Model file for the job. Use its own axes, mm. A direction names the side the tool comes from. Give positions to 0.01 mm unless a question says otherwise; leave off trailing zeros. Loops run counter-clockwise (first coordinate to the right, second up) from the corner with the lowest first, then second, coordinate; pieces in that order, holes last. Notation, with made-up numbers: (-34.5, 31.25) -> (24.5, 31.25) arc R12 cw to (24.5, 41.25) -> close; hole circle Ø4 at (38.5, 55). An arc over 180 degrees is marked (long way). Use CSV: the item, a comma, the result in double quotes. Start each with the question number.
(1) Flat gauge pins, fed straight in: pin 1 (1.8 mm diameter, centred on x = 0.5, z = -0.5, fed in from +Y); pin 2 (2 mm diameter, centred on y = 1, z = 1.5, fed in from +X); pin 3 (1 mm diameter, centred on y = 2, z = 1, fed in from -X). Where does each tip first touch, or does it go through?
(2) 3-axis set-ups, long thin cutter, end or side, ignore diameter. For faces 1 (the flat face through (2.39, 1.23, -1.36)), 2 (the cylindrical face through (1.01, 2.87, 2.45)): which of +Z, -Z, +X, -X, +Y, -Y reach the whole face in a straight line?
(3) Cut at A-A on y = 1.6. Write the cut outline in (x, z), then the cut area to 3 significant figures.
(4) Drill centre lines: probe 1 along X at (y, z) = (1.2, 0.1); probe 2 along Z at (x, y) = (-0.5, 1.1); probe 3 along Z at (x, y) = (1.25, 0.5). Where is each one in solid material? Low to high.
(5) Cut at C-C on y = 2.7. Write the cut outline in (x, z).
(6) Pull direction Z, two halves, no side cores. Call faces 3 (the flat face through (2.37, 1.234, 1.394)), 4 (the flat face through (0, 1, -2.75)), 5 (the flat face through (1.3, 0, -1.2)), 6 (the cylindrical face through (0.45, 1.97, 1.43)): pulls with the +Z half, pulls with the -Z half, needs draft (parallel to the pull), parting line crosses it, or undercut.
from build123d import *

# Parameters (mm, degrees)
SKETCH1_R           = 1.5
BOSS_EXTRUDE1_DEPTH = 4
FILLET1_R           = 0.1
CUT_EXTRUDE1_START  = -0.1
SKETCH3_R           = 1.8
SKETCH3_R_2         = 1.5
CUT_EXTRUDE1_DEPTH  = 0.1
FILLET2_R           = 0.1


with BuildPart() as part:
    # Sketch1 → Boss-Extrude1 (new body)
    with BuildSketch(Plane(origin=(0, 0, 0), x_dir=(1, 0, 0), z_dir=(0, 1, 0))):
        Polygon((1.58771324, -2.75), (3.175426481, 0), (1.58771324, 2.75), (-1.58771324, 2.75), (-3.175426481, 0), (-1.58771324, -2.75), align=None)
        with Locations(Location((0, 0, 0), (0, 0, 270))):
            Circle(SKETCH1_R, mode=Mode.SUBTRACT)
    extrude(amount=BOSS_EXTRUDE1_DEPTH)

    # Sketch2 → Cut-Revolve3 (revolve, cut)
    with BuildSketch(Plane(origin=(0, 0, 0), x_dir=(0, 0, -1), z_dir=(1, 0, 0))):
        with BuildLine():
            Line((-2.65, 3.25), (-2.65, 2.5))
            Line((-2.65, 2.5), (-5.25, 2.5))
            Line((-5.25, 2.5), (-5.25, 4))
            Line((-5.25, 4), (-5.25, 4.1))
            Line((-5.25, 4.1), (-1.9, 4.1))
            Line((-1.9, 4.1), (-1.9, 4))
            ThreePointArc((-1.9, 4), (-2.430330086, 3.780330086), (-2.65, 3.25))
        make_face()
    revolve(axis=Axis((0, 4, 0), (0, -1, 0)), mode=Mode.SUBTRACT)

    # Fillet1
    fillet1_edges = [part.edges().sort_by_distance(p)[0] for p in [
        (0, 0, -1.5),
        (-2.38156986, 2.5, 1.375),
        (2.38156986, 2.5, 1.375),
        (0, 2.5, 2.75),
        (-2.38156986, 2.5, -1.375),
        (0, 2.5, -2.75),
        (2.38156986, 2.5, -1.375),
        (-2.38156986, 0, 1.375),
        (-2.38156986, 0, -1.375),
        (0, 0, -2.75),
        (2.38156986, 0, -1.375),
        (2.38156986, 0, 1.375),
        (0, 0, 2.75),
    ]]
    fillet(fillet1_edges, radius=FILLET1_R - 0.0001)  # a hair under: the kernel refuses the full size

    # Sketch3 → Cut-Extrude1 (cut)
    with BuildSketch(Plane(origin=(0, 4, 0), x_dir=(1, 0, 0), z_dir=(0, 1, 0)).offset(CUT_EXTRUDE1_START)):
        with Locations(Location((0, 0, 0), (0, 0, 270))):
            Circle(SKETCH3_R)
        with Locations(Location((0, 0, 0), (0, 0, 270))):
            Circle(SKETCH3_R_2, mode=Mode.SUBTRACT)
    extrude(amount=CUT_EXTRUDE1_DEPTH, mode=Mode.SUBTRACT)

    # Fillet2
    fillet2_edges = [part.edges().sort_by_distance(p)[0] for p in [
        (0, 4, -1.8),
    ]]
    fillet(fillet2_edges, radius=FILLET2_R - 0.0001)  # a hair under: the kernel refuses the full size


solid = part.part
Check result:
1,pin 1,"y = 3.9"
1,pin 2,"x = 2.89"
1,pin 3,"x = -2.89"
2,face 1,"-Z, +X, +Y, -Y"
2,face 2,"+Y"
3,outline,"(-3.18, 0) -> (-1.59, -2.75) -> (1.59, -2.75) -> (3.18, 0) -> (1.59, 2.75) -> (-1.59, 2.75) -> close; hole circle Ø3 at (0, 0)"
3,area,"19.1 mm²"
4,probe 1,"-3.12 to -1.5, 1.5 to 3.12"
4,probe 2,"-2.75 to -1.41, 1.41 to 2.75"
4,probe 3,"-2.75 to -0.83, 0.83 to 2.75"
5,outline,"circle Ø5.3 at (0, 0); hole circle Ø3 at (0, 0)"
6,face 3,"pulls with the +Z half"
6,face 4,"pulls with the -Z half"
6,face 5,"needs draft"
6,face 6,"undercut"
